from build123d import *

# Parameters (mm, degrees)
SKETCH1_R           = 0.6
BOSS_EXTRUDE1_DEPTH = 1
SCALE1_SCALE        = 0.222222222
SCALE2_SCALE        = 1.25


with BuildPart() as part:
    # Sketch1 → Boss-Extrude1 (new body)
    with BuildSketch(Plane(origin=(19, 0, 0), x_dir=(0, 0, -1), z_dir=(1, 0, 0))):
        with BuildLine():
            Line((-1.082906578, 1.214226965), (-0.806260325, 1.444819657))
            ThreePointArc((-0.806260325, 1.444819657), (-0.157167996, 2.46989624), (-0.220083072, 3.681566388))
            ThreePointArc((-0.220083072, 3.681566388), (-20.449170804, -0.000103807), (-0.220095755, -3.681843689))
            ThreePointArc((-0.220095755, -3.681843689), (-0.157177378, -2.470170425), (-0.806270581, -1.44509051))
            Line((-0.806270581, -1.44509051), (-1.082193901, -1.213563353))
            ThreePointArc((-1.082193901, -1.213563353), (-3.437745717, -1.969386585), (-1.886859109, -3.896727719))
            ThreePointArc((-1.886859109, -3.896727719), (-18.999593972, -0.000121806), (-1.886859109, 3.896484108))
            ThreePointArc((-1.886859109, 3.896484108), (-3.437385157, 1.97013231), (-1.082906578, 1.214226965))
        make_face()
        with Locations((-2.00000003, -2.4)):
            Circle(SKETCH1_R, mode=Mode.SUBTRACT)
        with Locations((-2.00000003, 2.4)):
            Circle(SKETCH1_R, mode=Mode.SUBTRACT)
    extrude(amount=-BOSS_EXTRUDE1_DEPTH)


with BuildPart() as part_1:
    # Scale1: scaled about (18.5, -0.000178585, 9.916688181)
    add(part.part.scale(SCALE1_SCALE).moved(Location((14.388888889, -0.000138899, 7.712979696))))


with BuildPart() as part_2:
    # Scale2: scaled about (18.5, -0.000178585, 9.916688181)
    add(part_1.part.scale(SCALE2_SCALE).moved(Location((-4.625, 4.4646e-05, -2.479172045))))


solid = part_2.part
Build history of the part. All positions in model axes, mm. Coordinates: 2 decimals unless noted, no trailing zeros. Order: outer loops, then holes, each group sorted by start corner. A loop starts at its lowest first (then second) coordinate and runs counter-clockwise, first axis right, second up. Notation, with made-up numbers: (38, -26) - (43, -26) arc R19 ccw to (43, -12) - close; hole circle Ø5 at (9, -18). An arc over 180 degrees is marked (long way). Write each question's results on one line, items separated by ' | '. Start each with the question number.
Item 1: Wall check: probe 1 along Z at (x, y) = (18.4, 0.7); probe 2 along Y at (x, z) = (18.6, 11.1); probe 3 along Z at (x, y) = (18.4, 2). Give the ranges that are in metal, low to high. Write a range as [from, to].
Item 2: Band-saw the part on B-B on z = 8.2. Write the cut outline in (x, y), and give its area (3 significant figures).
Item 3: Band-saw the part on A-A on y = 2.3. Write the cut outline in (x, z), and give its area (3 significant figures).
Item 4: Band-saw the part on C-C on x = 18.5. Write the cut outline in (y, z).
Numbers:
1) probe 1: [7.2, 7.55], [7.88, 8.13], [12.34, 12.76] | probe 2: [-2.66, -2.21], [2.21, 2.66] | probe 3: [7.84, 8.44], [11.44, 12.04]
2) outline: (18.36, -2.32) - (18.64, -2.32) - (18.64, -1.8) - (18.36, -1.8) - close; (18.36, 1.8) - (18.64, 1.8) - (18.64, 2.32) - (18.36, 2.32) - close | area: 0.293 mm^2
3) outline: (18.36, 8.17) - (18.64, 8.17) - (18.64, 8.96) - (18.36, 8.96) - close; (18.36, 10.92) - (18.64, 10.92) - (18.64, 11.71) - (18.36, 11.71) - close | area: 0.439 mm^2
4) outline: (-1.08, 7.69) arc R2.5 cw (long way) to (1.08, 7.69) arc R0.42 ccw (long way) to (0.34, 7.46) - (0.4, 7.39) arc R0.56 ccw to (1.02, 7.22) arc R2.9 ccw (long way) to (-1.02, 7.22) arc R0.56 ccw to (-0.4, 7.39) - (-0.34, 7.46) arc R0.42 ccw (long way) to start; hole circle Ø0.33 at (-0.67, 7.72); hole circle Ø0.33 at (0.67, 7.72)
